Check sheet for the modelled part. Datum: model origin and axes. Units: mm. A direction names the side the tool comes from. Coordinates: 2 decimals unless noted, no trailing zeros. Write each loop counter-clockwise with the first axis right and the second up, starting at its lowest first coordinate (ties: lowest second). Pieces come first, ordered by that corner, then holes. Notation, with made-up numbers: M 26,54.25 L 74,54.25 A25 cw 74,75.25 Z; hole C 0,41.25 d10. An arc over 180 degrees is marked long. Answer as CSV lines item,"result". Start each with the question number.
1) Draft check along X on faces 1 (the flat face through (-28.4, -20.4, 3.5)), 2 (the flat face through (-32, -1.9, 0.8)), 3 (the flat face through (27, -19, 6.5)). Enter one of: +X half, -X half, draft (parallel to the pull), parting line (faces both ways), or undercut.
2) Section check B-B (y = -1). Record the cut outline in (x, z).
3) Section check D-D (z = 8). Record the cut outline in (x, y), and give its area (3 significant figures).
4) Access from +Z, -Z, +X, -X, +Y, -Y to the whole of each face (thin tool, end or side, straight path). Record for faces 4 (the flat face through (-28.451, -22.06, 8.137)), 5 (the flat face through (25, -23, 5)), 6 (the cylindrical face through (28.598, 18.514, 4.979)), 7 (the flat face through (28.5, 20.4, 3.5)), 8 (the flat face through (-28, -22.8, 5)).
5) Material ranges on L1, parallel to Z at x = -21, y = 21; L2, parallel to Y at x = -25.5, z = 2; L3, parallel to Y at x = 16, z = 0.5, recorded low to high. Write a range as [from, to].
6) Section check C-C (z = 4.5). Record the cut outline in (x, y) (3 decimals), and give its area (3 significant figures).
7) Section check A-A (x = 19). Record the cut outline in (y, z).
8) Go/stop test with flat-tipped pins: pin 1 Ø2 at (x, y) = (27, -18.5) entering from +Z; pin 2 Ø4 at (x, y) = (7, -15.5) entering from -Z. Record where each tip stops, or that it passes through.
from build123d import *

# Parameters (mm, degrees)
SKETCH_W        = 64
SKETCH_H        = 48
PAD_DEPTH       = 1
POCKET_DEPTH    = 1.001
SKETCH002_R     = 2.5
PAD001_DEPTH    = 2.5
SKETCH003_R     = 1.4
PAD002_DEPTH    = 3
SKETCH004_W     = 7
SKETCH004_H     = 2.7
PAD003_DEPTH    = 8
POCKET001_DEPTH = 225.010317


with BuildPart() as part:
    # Sketch → Pad (new body)
    with BuildSketch(Plane.XY):
        Rectangle(SKETCH_W, SKETCH_H)
    extrude(amount=PAD_DEPTH)

    # Sketch001 → Pocket (cut, through all)
    with BuildSketch(Plane.XY.offset(1)):
        Polygon((-27, 14), (-27, -14), (-22, -14), (-22, -19), (22, -19), (22, -14), (27, -14), (27, 14), (22, 14), (22, 19), (-22, 19), (-22, 14), align=None)
    extrude(amount=-POCKET_DEPTH, mode=Mode.SUBTRACT)

    # Sketch002 → Pad001 (new body)
    with BuildSketch(Plane.XY.offset(1)):
        with Locations((-27.305, 19.05)):
            Circle(SKETCH002_R)
        with Locations((-27.305, -19.05)):
            Circle(SKETCH002_R)
        with Locations((27.305, 19.05)):
            Circle(SKETCH002_R)
        with Locations((27.305, -19.05)):
            Circle(SKETCH002_R)
    extrude(amount=PAD001_DEPTH)

    # Sketch003 → Pad002 (new body)
    with BuildSketch(Plane.XY.offset(3.5)):
        with Locations((27.305, 19.05)):
            Circle(SKETCH003_R)
        with Locations((-27.305, -19.05)):
            Circle(SKETCH003_R)
        with Locations((27.305, -19.05)):
            Circle(SKETCH003_R)
        with Locations((-27.305, 19.05)):
            Circle(SKETCH003_R)
    extrude(amount=PAD002_DEPTH)

    # Sketch004 → Pad003 (new body)
    with BuildSketch(Plane.XY.offset(1)):
        with Locations((-28.5, -22.65)):
            Rectangle(SKETCH004_W, SKETCH004_H)
        with Locations((28.5, -22.65)):
            Rectangle(SKETCH004_W, SKETCH004_H)
        with Locations((28.5, 22.65)):
            Rectangle(SKETCH004_W, SKETCH004_H)
        with Locations((-28.5, 22.65)):
            Rectangle(SKETCH004_W, SKETCH004_H)
    extrude(amount=PAD003_DEPTH)

    # Sketch005 → Pocket001 (cut, through all)
    with BuildSketch(Plane.YZ.offset(32)):
        Polygon((-22.8, 9), (-21.3, 7.25), (-22.8, 5.5), (-22.8, 3.5), (-21.3, 3.5), (-21.2, 10), (-22.8, 10), align=None)
    pocket001 = extrude(amount=-POCKET001_DEPTH, mode=Mode.SUBTRACT)

    # Mirrored: Pocket001 across Sketch005 V_Axis
    add(pocket001.mirror(Plane(origin=(32, 0, 0), x_dir=(1, 0, 0), z_dir=(0, 1, 0))), mode=Mode.SUBTRACT)


solid = part.part
Results found:
1,face 1,"undercut"
1,face 2,"-X half"
1,face 3,"draft"
2,outline,"M -32,0 L -27,0 L -27,1 L -32,1 Z; M 27,0 L 32,0 L 32,1 L 27,1 Z"
3,outline,"M -32,-24 L -25,-24 L -25,-21.94 L -32,-21.94 Z; M -32,21.94 L -25,21.94 L -25,24 L -32,24 Z; M 25,-24 L 32,-24 L 32,-21.94 L 25,-21.94 Z; M 25,21.94 L 32,21.94 L 32,24 L 25,24 Z"
3,area,"57.6 mm2"
4,face 4,"+Z, +X, -X"
4,face 5,"+Z, -Y"
4,face 6,"+Z"
4,face 7,"none"
4,face 8,"+X, -X"
5,L1,"z = [0, 1]"
5,L2,"y = [-24, -21.3], [-20.78, -17.32], [17.32, 20.78], [21.3, 24]"
5,L3,"y = [-24, -19], [19, 24]"
6,outline,"M -32,-24 L -25,-24 L -25,-22.8 L -32,-22.8 Z; M -32,22.8 L -25,22.8 L -25,24 L -32,24 Z; C -27.305,-19.05 d2.8; C -27.305,19.05 d2.8; M 25,-24 L 32,-24 L 32,-22.8 L 25,-22.8 Z; M 25,22.8 L 32,22.8 L 32,24 L 25,24 Z; C 27.305,-19.05 d2.8; C 27.305,19.05 d2.8"
6,area,"58.2 mm2"
7,outline,"M -24,0 L -19,0 L -19,1 L -24,1 Z; M 19,0 L 24,0 L 24,1 L 19,1 Z"
8,pin 1,"stops at z = 6.5"
8,pin 2,"passes through"
